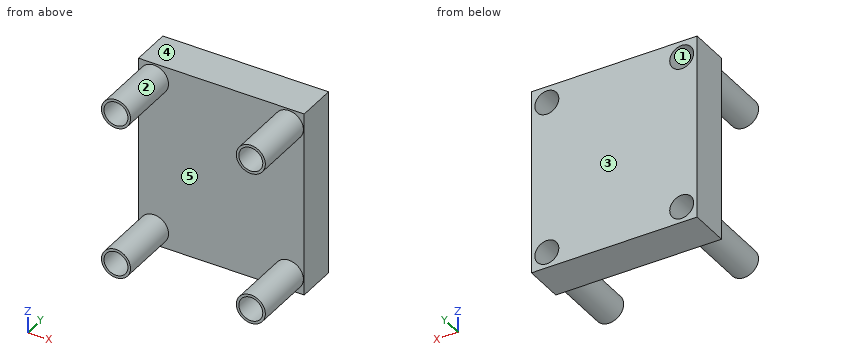
```python
from build123d import *

# Parameters (mm, degrees)
SKETCH1_W               = 22.733
SKETCH1_H               = 25.5016
BOSS_EXTRUDE1_DEPTH     = 5.4864
SKETCH2_R               = 1.9939
SKETCH2_R_2             = 1.642387972
BOSS_EXTRUDE2_DEPTH     = 8.5852
SKETCH5_R               = 1.642387972
CUT_EXTRUDE1_DEPTH      = 1
CUT_EXTRUDE1_DEPTH_BACK = 15.0716


with BuildPart() as part:
    # Sketch1 → Boss-Extrude1 (new body)
    with BuildSketch(Plane(origin=(0, 0, 0), x_dir=(1, 0, 0), z_dir=(0, 1, 0))):
        with Locations((-22.674199551, -11.077689686)):
            Rectangle(SKETCH1_W, SKETCH1_H)
    extrude(amount=BOSS_EXTRUDE1_DEPTH)

    # Sketch2 → Boss-Extrude2 (add)
    with BuildSketch(Plane.XZ):
        with Locations((-31.918497565, 21.596793601)):
            Circle(SKETCH2_R)
        with Locations((-31.918497565, 21.596793601)):
            Circle(SKETCH2_R_2, mode=Mode.SUBTRACT)
        with Locations((-13.414259747, 21.596793601)):
            Circle(SKETCH2_R)
        with Locations((-13.414259747, 21.596793601)):
            Circle(SKETCH2_R_2, mode=Mode.SUBTRACT)
        with Locations((-31.918497565, 0.511660399)):
            Circle(SKETCH2_R)
        with Locations((-31.918497565, 0.511660399)):
            Circle(SKETCH2_R_2, mode=Mode.SUBTRACT)
        with Locations((-13.414259747, 0.511660399)):
            Circle(SKETCH2_R)
        with Locations((-13.414259747, 0.511660399)):
            Circle(SKETCH2_R_2, mode=Mode.SUBTRACT)
    extrude(amount=BOSS_EXTRUDE2_DEPTH)

    # Sketch5 → Cut-Extrude1 (cut, two sides)
    with BuildSketch(Plane(origin=(0, 5.4864, 0), x_dir=(1, 0, 0), z_dir=(0, 1, 0))) as cut_extrude1_sk:
        with Locations((-31.918497565, -0.511660399)):
            Circle(SKETCH5_R)
        with Locations((-13.414259747, -0.511660399)):
            Circle(SKETCH5_R)
        with Locations((-13.414259747, -21.596793601)):
            Circle(SKETCH5_R)
        with Locations((-31.918497565, -21.596793601)):
            Circle(SKETCH5_R)
    extrude(amount=CUT_EXTRUDE1_DEPTH, mode=Mode.SUBTRACT)
    extrude(cut_extrude1_sk.sketch, amount=-CUT_EXTRUDE1_DEPTH_BACK, mode=Mode.SUBTRACT)


solid = part.part
```
Work out the finished part from the listing and answer in its coordinate system (mm). Face numbers are marked on the shaded views. A direction names the side the tool comes from. Give positions to 0.01 mm unless a question says otherwise; leave off trailing zeros. Write each loop counter-clockwise with the first axis right and the second up, starting at its lowest first coordinate (ties: lowest second). Pieces come first, ordered by that corner, then holes. Notation, with made-up numbers: (47, -14.5) - (100, -14.5) arc R16 cw to (100, 11.5) - close; hole circle Ø10 at (-16.75, 18). An arc over 180 degrees is marked (long way). Use one line per item in the form item = value.
1. A cutting plane is placed at D-D (z = 19). Write down the section's boundary in (x, y).
Filled in:
outline = (-34.04, 0) - (-11.31, 0) - (-11.31, 5.49) - (-34.04, 5.49) - close
2. A cutting plane is placed at A-A (y = -1.25). Write down the section's boundary in (x, z), and give its area (3 significant figures).
Filled in:
outline = circle Ø3.99 at (-31.92, 0.51); circle Ø3.99 at (-31.92, 21.6); circle Ø3.99 at (-13.41, 0.51); circle Ø3.99 at (-13.41, 21.6); hole circle Ø3.28 at (-31.92, 0.51); hole circle Ø3.28 at (-31.92, 21.6); hole circle Ø3.28 at (-13.41, 0.51); hole circle Ø3.28 at (-13.41, 21.6)
area = 16.1 mm^2
3. Each of these flat-tipped pins is pushed along its axis until it touches: pin 1 Ø4 at (x, z) = (-31.92, 0.51) entering from -Y; pin 2 Ø4 at (y, z) = (-6.5, 18) entering from +X. Where does it stop, or does it pass through?
Filled in:
pin_1 = -8.59
pin_2 = -12.22
4. Consider L1, parallel to X at y = -0.25, z = 20.5; L2, parallel to Z at x = -30.5, y = -7.5; L3, parallel to Z at x = -13, y = -1.5. Determine where each line is inside the solid, lowest interval first.
Filled in:
L1 = -33.58 to -33.14, -30.7 to -30.25, -15.08 to -14.64, -12.19 to -11.75
L2 = -0.89 to -0.32, 1.34 to 1.91, 20.2 to 20.77, 22.42 to 23
L3 = -1.44 to -1.08, 2.1 to 2.46, 19.65 to 20.01, 23.19 to 23.55
5. A cutting plane is placed at B-B (y = 3.25). Write down the section's boundary in (x, z), and give its area (3 significant figures).
Filled in:
outline = (-34.04, -1.67) - (-11.31, -1.67) - (-11.31, 23.83) - (-34.04, 23.83) - close; hole circle Ø3.28 at (-31.92, 0.51); hole circle Ø3.28 at (-31.92, 21.6); hole circle Ø3.28 at (-13.41, 0.51); hole circle Ø3.28 at (-13.41, 21.6)
area = 546 mm^2
6. For the marked faces 1 and 2, determine the directions among +Z, -Z, +X, -X, +Y, -Y from which every point of the face is accessible in a straight line to the end or side of a thin tool.
Filled in:
face_1 = +Y, -Y
face_2 = -Y
7. A cutting plane is placed at C-C (x = -32.25). Write down the section's boundary in (y, z).
Filled in:
outline = (-8.59, -1.45) - (0, -1.45) - (0, -1.67) - (5.49, -1.67) - (5.49, -1.1) - (-8.59, -1.1) - close; (-8.59, 2.12) - (5.49, 2.12) - (5.49, 19.99) - (-8.59, 19.99) - (-8.59, 19.63) - (0, 19.63) - (0, 2.48) - (-8.59, 2.48) - close; (-8.59, 23.21) - (5.49, 23.21) - (5.49, 23.83) - (0, 23.83) - (0, 23.56) - (-8.59, 23.56) - close
8. Determine the mould class of the marked faces 3, 4 and 5 for opening direction Y: released by +Y, released by -Y, zero draft, split by the parting line, or undercut.
Filled in:
face_3 = released by +Y
face_4 = zero draft
face_5 = released by -Y
